The listing builds one solid part. Answer for the finished solid, in the listing's coordinates (mm). A direction names the side the tool comes from. Give positions to 0.01 mm unless a question says otherwise; leave off trailing zeros. Write each loop counter-clockwise with the first axis right and the second up, starting at its lowest first coordinate (ties: lowest second). Pieces come first, ordered by that corner, then holes. Notation, with made-up numbers: (46, -31) - (54, -31) arc R27 cw to (54, -6) - close; hole circle Ø8 at (66, 11). An arc over 180 degrees is marked (long way). One line per question, with ' | ' between items. Start each with the question number.
1. A cutting plane is placed at B-B (x = -119). Determine the outline of the cut face in (y, z).
2. The mould has two halves that part along X. Classify faces 4 (the face through (201.106, 6.439, -110.342)), 5 (the face through (49, 19.05, 52)), 6 (the face through (302.693, 6, 59)): +X half, -X half, draft (parallel to the pull), parting line (faces both ways), or undercut.
3. Given P1, Ø12, axis at x = -151, z = -79.5, coming from the +Y side; P2, Ø3, axis at y = 15, z = 59.5, coming from the -X side; P3, Ø5, axis at y = 17.5, z = 148.5, coming from the +X side, each flat-ended and moving along its own axis, determine where each tip first touches the part or whether it passes through.
4. Find the intervals of material crossed by L1, parallel to Z at x = 222.5, y = 3.75; L2, parallel to Z at x = 220, y = 11; L3, parallel to Y at x = 262.5, z = -161.5, in increasing order. Write a range as from..to.
5. A cutting plane is placed at D-D (x = 182). Determine the outline of the cut face in (y, z), then the cut area to 3 significant figures.
6. For faces 1 (the face through (45, 7, 309.316)), 2 (the face through (-83, 12.7, 59)), 3 (the face through (184, 12.7, 59)), determine the directions among +Z, -Z, +X, -X, +Y, -Y from which every point of the face is accessible in a straight line to the end or side of a thin tool.
7. A cutting plane is placed at A-A (z = -79). Determine the outline of the cut face in (x, y).
8. A cutting plane is placed at C-C (z = 227). Determine the outline of the cut face in (x, y), then the cut area to 3 significant figures.
Autodesk Inventor part; units mm, degrees
ref_plane "YZ Plane" through (0, 0, 0) normal (1, 0, 0) x (0, 1, 0)
ref_plane "XZ Plane" through (0, 0, 0) normal (0, 1, 0) x (-1, 0, 0)
ref_plane "XY Plane" through (0, 0, 0) normal (0, 0, 1) x (1, 0, 0)
sketch "Sketch1" plane through (0, 0, 0) normal (0, 0, 1) x (1, 0, 0)
  point P0 (0, 0)
sketch "Sketch2" plane through (0, 0, 0) normal (0, 1, 0) x (-1, 0, 0)
  line L0 (205.3066, 309.3165) -> (-302.6934, 309.3165)
  line L1 (-302.6934, 309.3165) -> (-302.6934, -198.6835)
  line L2 (-302.6934, -198.6835) -> (205.3066, -198.6835)
  line L3 (205.3066, -198.6835) -> (205.3066, 309.3165)
  point P0 (0, 0)
  dimension "d0" = 508
  dimension "d1" = 508
extrude "Extrusion1" add sketch "Sketch2" along normal blind 12.7
sketch "Sketch3" plane through (0, 12.7, 0) normal (0, 1, 0) x (1, 0, 0)
  line L0 (-205.3066, -309.3165) -> (-116.4066, -309.3165)
  line L1 (-116.4066, -309.3165) -> (-116.4066, -220.4165)
  line L2 (-116.4066, -220.4165) -> (-205.3066, -220.4165)
  line L3 (-205.3066, -220.4165) -> (-205.3066, -309.3165)
  line L4 (-205.3066, 198.6835) -> (-116.4066, 198.6835)
  line L5 (-116.4066, 198.6835) -> (-116.4066, 109.7835)
  line L6 (-116.4066, 109.7835) -> (-205.3066, 109.7835)
  line L7 (-205.3066, 109.7835) -> (-205.3066, 198.6835)
  line L8 (302.6934, 198.6835) -> (213.7934, 198.6835)
  line L9 (213.7934, 198.6835) -> (213.7934, 109.7835)
  line L10 (213.7934, 109.7835) -> (302.6934, 109.7835)
  line L11 (302.6934, 109.7835) -> (302.6934, 198.6835)
  line L12 (302.6934, -309.3165) -> (213.7934, -309.3165)
  line L13 (213.7934, -309.3165) -> (213.7934, -220.4165)
  line L14 (213.7934, -220.4165) -> (302.6934, -220.4165)
  line L15 (302.6934, -220.4165) -> (302.6934, -309.3165)
  circle A0 centre (-116.4066, -220.4165) radius 12.7
  circle A1 centre (-116.4066, 109.7835) radius 12.7
  circle A2 centre (213.7934, 109.7835) radius 12.7
  circle A3 centre (213.7934, -220.4165) radius 12.7
  point P0 (0, 0)
  dimension "d4" = 88.9
  dimension "d5" = 88.9
  dimension "d6" = 88.9
  dimension "d7" = 88.9
  dimension "d8" = 88.9
  dimension "d9" = 88.9
  dimension "d10" = 88.9
  dimension "d11" = 88.9
  dimension "d12" = 25.4
  dimension "d13" = 25.4
  dimension "d14" = 25.4
  dimension "d15" = 25.4
extrude "Extrusion2" cut sketch "Sketch3" against normal blind 12.7 contours A0 L2 L1 | L1 L2 A0 | A1 L6 L5 | L5 L6 A1 | A2 L10 L9 | L9 L10 A2 | A3 L14 L13 | L13 L14 A3
sketch "Sketch4" plane through (0, 12.7, 0) normal (0, 1, 0) x (1, 0, 0)
  line L0 (302.6934, -309.3165) -> (-205.3066, -309.3165)
  line L1 (-205.3066, 198.6835) -> (302.6934, 198.6835)
  line L2 (302.6934, 198.6835) -> (48.6934, 198.6835)
  line L3 (48.6934, 198.6835) -> (74.0934, 198.6835)
  line L4 (74.0934, 198.6835) -> (61.3934, 198.6835)
  line L5 (61.3934, 198.6835) -> (35.9934, 198.6835)
  line L6 (35.9934, 198.6835) -> (35.9934, -309.3165)
  line L7 (35.9934, -309.3165) -> (61.3934, -309.3165)
  line L8 (61.3934, -309.3165) -> (61.3934, 198.6835)
  line L9 (61.3934, 198.6835) -> (35.9934, 198.6835)
  line L10 (35.9934, 198.6835) -> (35.9934, -309.3165)
  point P0 (0, 0)
  dimension "d18" = 254
  dimension "d19" = 25.4
  dimension "d20" = 12.7
  dimension "d21" = 25.4
extrude "Extrusion3" add sketch "Sketch4" along normal blind 6.35
properties part number "base"
Determined:
1) outline: (0, -198.68) - (12.7, -198.68) - (12.7, -122.22) - (0, -122.22) - close; (0, -97.35) - (12.7, -97.35) - (12.7, 207.98) - (0, 207.98) - close; (0, 232.85) - (12.7, 232.85) - (12.7, 309.32) - (0, 309.32) - close
2) face 4: undercut | face 5: draft | face 6: +X half
3) P1: y = 12.7 | P2: x = 35.99 | P3: x = 61.39
4) L1: -198.68..-119.03, -100.54..211.17, 229.66..309.32 | L2: -198.68..-120.86, -98.7..209.34, 231.5..309.32 | L3: 0..12.7
5) outline: (0, -198.68) - (12.7, -198.68) - (12.7, 309.32) - (0, 309.32) - close | area: 6,450 mm2
6) face 1: +Z, +X, -X, +Y, -Y | face 2: +Z, -Z, -X, +Y | face 3: +Z, -Z, +X, +Y
7) outline: (-205.31, 0) - (302.69, 0) - (302.69, 12.7) - (61.39, 12.7) - (61.39, 19.05) - (35.99, 19.05) - (35.99, 12.7) - (-205.31, 12.7) - close
8) outline: (-205.31, 0) - (-127.27, 0) - (-127.27, 12.7) - (-205.31, 12.7) - close; (-105.55, 0) - (202.93, 0) - (202.93, 12.7) - (61.39, 12.7) - (61.39, 19.05) - (35.99, 19.05) - (35.99, 12.7) - (-105.55, 12.7) - close; (224.65, 0) - (302.69, 0) - (302.69, 12.7) - (224.65, 12.7) - close | area: 6,060 mm2
